Design review of the part built by this model. Coordinates are the model's own, in mm. A direction names the side the tool comes from. Coordinates: 2 decimals unless noted, no trailing zeros. Write each loop counter-clockwise with the first axis right and the second up, starting at its lowest first coordinate (ties: lowest second). Pieces come first, ordered by that corner, then holes. Notation, with made-up numbers: (56.25, 47.25) -> (108.25, 47.25) arc R11 ccw to (108.25, 57.25) -> close; hole circle Ø8 at (6.25, -13.5). An arc over 180 degrees is marked (long way). One line per question, with ' | ' between items. Start each with the question number.
Q1. Wall thickness on probe 1 along Z at (x, y) = (30.48, 4); probe 2 along X at (y, z) = (3.45, 0): over which ranges is each line inside the solid? List them lowest first.
Q2. Add section D-D on z = 0. State the section outline as (x, y) points.
Q3. Add section A-A on x = -30.48. State the section outline as (y, z) points, and give its area (3 significant figures).
Q4. Add section C-C on x = 0. State the section outline as (y, z) points, and give its area (3 significant figures).
Q5. Add section B-B on z = -30.48. State the section outline as (x, y) points, and give its area (3 significant figures).
Q6. Draft analysis for pull direction X (two halves, no side actions). For faces 1 (the flat face through (0, 3, 38.1)), 2 (the cylindrical face through (-2.75, 3.83, 12.4)), 3 (the cylindrical face through (36.572, 2.504, 36.651)), state which applies: pulls with the +X half, pulls with the -X half, needs draft (parallel to the pull), parting line crosses it, or undercut.
Q7. For faces 4 (the flat face through (-38.1, 3, 0)), 5 (the flat face through (-6, 2.54, -9)), list the 3-axis set-ups (+Z, -Z, +X, -X, +Y, -Y) from which the entire face can be reached by the end or side of a thin tool; tool diameter is ignored.
from build123d import *

# Parameters (mm, degrees)
SKETCH1_R           = 10.16
SKETCH1_R_2         = 2.54
BOSS_EXTRUDE1_DEPTH = 5.08
SKETCH2_R           = 12.7
CUT_EXTRUDE1_DEPTH  = 2.54


with BuildPart() as part:
    # Sketch1 → Boss-Extrude1 (new body)
    with BuildSketch(Plane(origin=(0, 0, 0), x_dir=(1, 0, 0), z_dir=(0, 1, 0))):
        with BuildLine():
            Line((-33.02, -38.1), (33.02, -38.1))
            ThreePointArc((33.02, -38.1), (36.612102448, -36.612102448), (38.1, -33.02))
            Line((38.1, -33.02), (38.1, 33.02))
            ThreePointArc((38.1, 33.02), (36.612102448, 36.612102448), (33.02, 38.1))
            Line((33.02, 38.1), (-33.02, 38.1))
            ThreePointArc((-33.02, 38.1), (-36.612102448, 36.612102448), (-38.1, 33.02))
            Line((-38.1, 33.02), (-38.1, -33.02))
            ThreePointArc((-38.1, -33.02), (-36.612102448, -36.612102448), (-33.02, -38.1))
        make_face()
        Circle(SKETCH1_R, mode=Mode.SUBTRACT)
        with Locations((-30.48, 30.48)):
            Circle(SKETCH1_R_2, mode=Mode.SUBTRACT)
        with Locations((30.48, 30.48)):
            Circle(SKETCH1_R_2, mode=Mode.SUBTRACT)
        with Locations((30.48, -30.48)):
            Circle(SKETCH1_R_2, mode=Mode.SUBTRACT)
        with Locations((-30.48, -30.48)):
            Circle(SKETCH1_R_2, mode=Mode.SUBTRACT)
    extrude(amount=BOSS_EXTRUDE1_DEPTH)

    # Sketch2 → Cut-Extrude1 (cut)
    with BuildSketch(Plane(origin=(0, 5.08, 0), x_dir=(1, 0, 0), z_dir=(0, 1, 0))):
        Circle(SKETCH2_R)
    extrude(amount=-CUT_EXTRUDE1_DEPTH, mode=Mode.SUBTRACT)


solid = part.part
Output values:
1) probe 1: z = -38.1 to -33.02, -27.94 to 27.94, 33.02 to 38.1 | probe 2: x = -38.1 to -12.7, 12.7 to 38.1
2) outline: (-38.1, 0) -> (-10.16, 0) -> (-10.16, 2.54) -> (-12.7, 2.54) -> (-12.7, 5.08) -> (-38.1, 5.08) -> close; (10.16, 0) -> (38.1, 0) -> (38.1, 5.08) -> (12.7, 5.08) -> (12.7, 2.54) -> (10.16, 2.54) -> close
3) outline: (0, -38.1) -> (5.08, -38.1) -> (5.08, -33.02) -> (0, -33.02) -> close; (0, -27.94) -> (5.08, -27.94) -> (5.08, 27.94) -> (0, 27.94) -> close; (0, 33.02) -> (5.08, 33.02) -> (5.08, 38.1) -> (0, 38.1) -> close | area: 335 mm2
4) outline: (0, -38.1) -> (5.08, -38.1) -> (5.08, -12.7) -> (2.54, -12.7) -> (2.54, -10.16) -> (0, -10.16) -> close; (0, 10.16) -> (2.54, 10.16) -> (2.54, 12.7) -> (5.08, 12.7) -> (5.08, 38.1) -> (0, 38.1) -> close | area: 271 mm2
5) outline: (-38.1, 0) -> (-33.02, 0) -> (-33.02, 5.08) -> (-38.1, 5.08) -> close; (-27.94, 0) -> (27.94, 0) -> (27.94, 5.08) -> (-27.94, 5.08) -> close; (33.02, 0) -> (38.1, 0) -> (38.1, 5.08) -> (33.02, 5.08) -> close | area: 335 mm2
6) face 1: needs draft | face 2: undercut | face 3: pulls with the +X half
7) face 4: +Z, -Z, -X, +Y, -Y | face 5: +Y
